from build123d import *

# Parameters (mm, degrees)
SKETCH_1_R                       = 4.5
MOVING_POST_A_DEPTH              = 8
SKETCH_2_R                       = 58
CUP_PLATE_D116_T4_DEPTH          = 4
SKETCH_3_R                       = 4.5
MOVING_POST_B_DEPTH              = 8
SKETCH_4_R                       = 58
SKETCH_4_R_2                     = 55.5
DRIP_SKIRT_OD116_ID111_H10_DEPTH = 10
SKETCH_5_R                       = 2.15
M4_MOVING_MOUNT_CLEARANCE_DEPTH  = 8
CUP_TOP_OUTER_ROUND_R2_R         = 2


with BuildPart() as part:
    # 草图1 → Moving_post_A (new body)
    with BuildSketch(Plane(origin=(0, 0, 0), x_dir=(1, 0, 0), z_dir=(0, 1, 0))):
        with Locations(Location((-22, 0, 0), (0, 0, 270))):
            Circle(SKETCH_1_R)
    extrude(amount=MOVING_POST_A_DEPTH)

    # 草图2 → Cup_plate_D116_T4 (add)
    with BuildSketch(Plane(origin=(0, 0, 0), x_dir=(1, 0, 0), z_dir=(0, 1, 0))):
        with Locations(Location((0, 0, 0), (0, 0, 270))):
            Circle(SKETCH_2_R)
    extrude(amount=CUP_PLATE_D116_T4_DEPTH)

    # 草图3 → Moving_post_B (add)
    with BuildSketch(Plane(origin=(0, 0, 0), x_dir=(1, 0, 0), z_dir=(0, 1, 0))):
        with Locations(Location((-32, 0, 0), (0, 0, 270))):
            Circle(SKETCH_3_R)
    extrude(amount=MOVING_POST_B_DEPTH)

    # 草图4 → Drip_skirt_OD116_ID111_H10 (add)
    with BuildSketch(Plane(origin=(0, 0, 0), x_dir=(1, 0, 0), z_dir=(0, 1, 0))):
        with Locations(Location((0, 0, 0), (0, 0, 270))):
            Circle(SKETCH_4_R)
        with Locations(Location((0, 0, 0), (0, 0, 270))):
            Circle(SKETCH_4_R_2, mode=Mode.SUBTRACT)
    extrude(amount=DRIP_SKIRT_OD116_ID111_H10_DEPTH)

    # 草图5 → M4_moving_mount_clearance (cut)
    with BuildSketch(Plane(origin=(0, 0, 0), x_dir=(1, 0, 0), z_dir=(0, 1, 0))):
        with Locations(Location((-22, 0, 0), (0, 0, 270))):
            Circle(SKETCH_5_R)
        with Locations(Location((-32, 0, 0), (0, 0, 270))):
            Circle(SKETCH_5_R)
    extrude(amount=M4_MOVING_MOUNT_CLEARANCE_DEPTH, mode=Mode.SUBTRACT)

    # Cup_top_outer_round_R2
    cup_top_outer_round_r2_edges = [part.edges().sort_by_distance(p)[0] for p in [
        (0, 10, -58),
    ]]
    fillet(cup_top_outer_round_r2_edges, radius=CUP_TOP_OUTER_ROUND_R2_R)


solid = part.part
Check sheet for the modelled part. Datum: model origin and axes. Units: mm. A direction names the side the tool comes from. Coordinates: 2 decimals unless noted, no trailing zeros. Write each loop counter-clockwise with the first axis right and the second up, starting at its lowest first coordinate (ties: lowest second). Pieces come first, ordered by that corner, then holes.
Item 1: Cross-section at A-A on y = 5.5. Record the boundary of the cut face in (x, z), then the cut area to 3 significant figures.
Numbers:
outline: circle Ø116 at (0, 0); circle Ø9 at (-32, 0); circle Ø9 at (-22, 0); hole circle Ø111 at (0, 0); hole circle Ø4.3 at (-32, 0); hole circle Ø4.3 at (-22, 0)
area: 990 mm2
Item 2: Scan lines: probe 1 along X at (y, z) = (3.75, 0); probe 2 along X at (y, z) = (8.05, 0); probe 3 along Y at (x, z) = (26, 41). Record each from-to range of solid material in increasing order.
Numbers:
probe 1: x = -58 to -34.15, -29.85 to -24.15, -19.85 to 58
probe 2: x = -58 to -55.5, 55.5 to 58
probe 3: y = 0 to 4
Item 3: Cross-section at C-C on x = 0. Record the boundary of the cut face in (y, z), then the cut area to 3 significant figures.
Numbers:
outline: (0, -58) - (8, -58) arc R2 ccw to (10, -56) - (10, -55.5) - (4, -55.5) - (4, 55.5) - (10, 55.5) - (10, 56) arc R2 ccw to (8, 58) - (0, 58) - close
area: 492 mm2
Item 4: Depth check by flat-ended pin: pin 1 Ø6 at (y, z) = (6.5, 39.5) entering from +X; pin 2 Ø12 at (x, z) = (26, -32) entering from +Y; pin 3 Ø2.5 at (x, z) = (-30.5, 0.5) entering from +Y. Enter the tip coordinate at first touch or a pass-through.
Numbers:
pin 1: stops at x = 45.07
pin 2: stops at y = 4
pin 3: stops at y = 8
Item 5: Mould release check, pull along Z, two halves, no side actions. Record for faces 1 (the face through (-24.1, 3.94, -0.47)), 2 (the face through (-22.21, 3.94, 53.58)), 3 (the face through (1, 0, -1)): released by +Z, released by -Z, zero draft, split by the parting line, or undercut.
Numbers:
face 1: undercut
face 2: split by the parting line
face 3: zero draft
Item 6: Cross-section at B-B on z = 0. Record the boundary of the cut face in (x, y).
Numbers:
outline: (-58, 0) - (-34.15, 0) - (-34.15, 8) - (-36.5, 8) - (-36.5, 4) - (-55.5, 4) - (-55.5, 10) - (-56, 10) arc R2 ccw to (-58, 8) - close; (-29.85, 0) - (-24.15, 0) - (-24.15, 8) - (-26.5, 8) - (-26.5, 4) - (-27.5, 4) - (-27.5, 8) - (-29.85, 8) - close; (-19.85, 0) - (58, 0) - (58, 8) arc R2 ccw to (56, 10) - (55.5, 10) - (55.5, 4) - (-17.5, 4) - (-17.5, 8) - (-19.85, 8) - close
Item 7: Access from +Z, -Z, +X, -X, +Y, -Y to the whole of each face (thin tool, end or side, straight path). Record for faces 4 (the face through (1, 4, -1)), 5 (the face through (12.7, 10, -54.2)).
Numbers:
face 4: +Y
face 5: +Z, -Z, +X, -X, +Y
